Geometry: final body of the model. Coordinates: model frame, mm. Give positions to 0.01 mm unless a question says otherwise; leave off trailing zeros. Order: outer loops, then holes, each group sorted by start corner. A loop starts at its lowest first (then second) coordinate and runs counter-clockwise, first axis right, second up. Notation, with made-up numbers: (87, 80) -> (95, 80) arc R21 ccw to (95, 102) -> close; hole circle Ø11 at (-15, 81). An arc over 180 degrees is marked (long way). One line per question, with ' | ' between items. Start each with the question number.
(1) Section A-A (z = -38.25). Return loops of the section in (x, y) (3 decimals).
(2) Section C-C (y = -0.5). Return loops of the section in (x, z) (3 decimals).
(3) Section B-B (x = -7). Return loops of the section in (y, z) (3 decimals), then the cut area to 3 significant figures.
(4) First-contact query: pin 1 Ø1 at (y, z) = (1, -28.5) entering from +X (3 decimals); pin 2 Ø1.9 at (x, y) = (9, 1) entering from -Z. Flat tips, straight axial feed; report the tip coordinate or a pass-through.
(5) Ray query, L1, parallel to Z at x = 8.75, y = 1; L2, parallel to X at y = 0.25, z = -38.25 (3 decimals); L3, parallel to X at y = 2.5, z = -28.5 (3 decimals). Return the intervals inside material, ascending.
```python
from build123d import *

# Parameters (mm, degrees)
SKETCH1_R           = 7
BOSS_EXTRUDE1_DEPTH = 3.175


with BuildPart() as part:
    # Sketch1 → Boss-Extrude1 (new, symmetric)
    with BuildSketch(Plane(origin=(0, 0, 0), x_dir=(1, 0, 0), z_dir=(0, 1, 0))):
        Polygon((-13.175, 47.5), (-13.175, -47.5), (13.175, -47.5), (13.175, -37.5), (6.825, -37.5), (6.825, -7.5), (13.175, -7.5), (13.175, 2.5), (6.825, 2.5), (6.825, 32.5), (13.175, 32.5), (13.175, 42.5), (6.825, 42.5), (6.825, 47.5), align=None)
        with Locations(Location((-3.175, 38.25, 0), (0, 0, 270))):
            Circle(SKETCH1_R, mode=Mode.SUBTRACT)
    extrude(amount=BOSS_EXTRUDE1_DEPTH, both=True)


solid = part.part
```
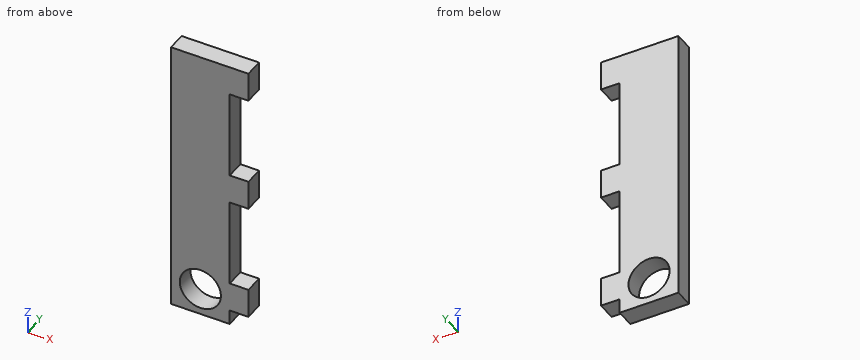
Response:
1) outline: (-13.175, -3.175) -> (-10.175, -3.175) -> (-10.175, 3.175) -> (-13.175, 3.175) -> close; (3.825, -3.175) -> (13.175, -3.175) -> (13.175, 3.175) -> (3.825, 3.175) -> close
2) outline: (-13.175, -47.5) -> (6.825, -47.5) -> (6.825, -42.5) -> (13.175, -42.5) -> (13.175, -32.5) -> (6.825, -32.5) -> (6.825, -2.5) -> (13.175, -2.5) -> (13.175, 7.5) -> (6.825, 7.5) -> (6.825, 37.5) -> (13.175, 37.5) -> (13.175, 47.5) -> (-13.175, 47.5) -> close; hole circle Ø14 at (-3.175, -38.25)
3) outline: (-3.175, -47.5) -> (3.175, -47.5) -> (3.175, -44.113) -> (-3.175, -44.113) -> close; (-3.175, -32.387) -> (3.175, -32.387) -> (3.175, 47.5) -> (-3.175, 47.5) -> close | area: 529 mm^2
4) pin 1: stops at x = 6.825 | pin 2: stops at z = -42.5
5) L1: z = -42.5 to -32.5, -2.5 to 7.5, 37.5 to 47.5 | L2: x = -13.175 to -10.175, 3.825 to 13.175 | L3: x = -13.175 to 6.825
